CAD build for the part. Positions are in the model's coordinates, mm. Face numbers are marked on the shaded views. A direction names the side the tool comes from. Give positions to 0.01 mm unless a question says otherwise; leave off trailing zeros. Order: outer loops, then holes, each group sorted by start corner. A loop starts at its lowest first (then second) coordinate and runs counter-clockwise, first axis right, second up.
from build123d import *

# Parameters (mm, degrees)
F0_W     = 30
F0_H     = 50
F0_W_2   = 24
F0_H_2   = 44
F1_DEPTH = 250
F3_D     = 5.5
F5_D     = 10
F5_DEPTH = 5


with BuildPart() as f1:
    # F0 (on Top) → F1 (new body)
    with BuildSketch(Plane.XY):
        with Locations((15, 25)):
            Rectangle(F0_W, F0_H)
        with Locations((15, 25)):
            Rectangle(F0_W_2, F0_H_2, mode=Mode.SUBTRACT)
    extrude(amount=F1_DEPTH)

    # F3 (through all)
    with Locations(Plane(origin=(0, 0, 0), x_dir=(0, -1, 0), z_dir=(-1, 0, 0))):
        with Locations((-25, 220)):
            Hole(F3_D / 2)

    # F5
    with Locations(Plane.YZ.offset(30)):
        with Locations((25, 220)):
            Hole(F5_D / 2, depth=F5_DEPTH)


solid = f1.part
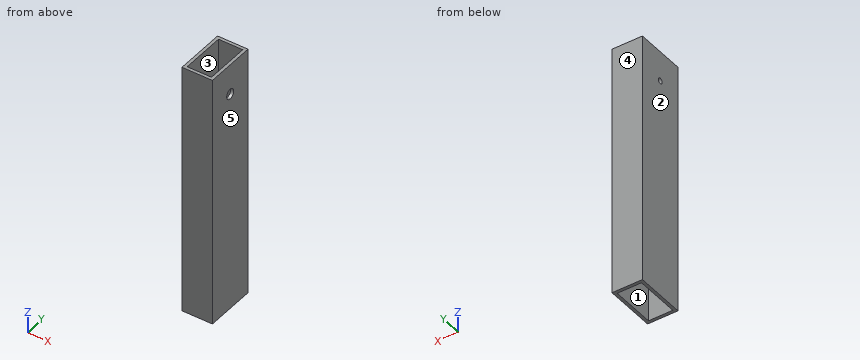
1. 3-axis set-ups, long thin cutter, end or side, ignore diameter. For the marked faces 1 and 2: which of +Z, -Z, +X, -X, +Y, -Y reach the whole face in a straight line?
2. Saw through at B-B on y = 44. Give the cut face in (x, z).
3. Saw through at A-A on x = 23.75. Give the cut face in (y, z), plus the area to 3 significant figures.
4. Mould opens along X. For the marked faces 3, 4 and 5 say: released by +X, released by -X, zero draft, split by the parting line, or undercut.
5. Saw through at C-C on z = 220. Give the cut face in (x, y), plus the area to 4 significant figures.
6. Wall check: line 1 (Z direction, x = 27.8, y = 25); line 2 (Y direction, x = 7.5, z = 87); line 3 (Z direction, x = 2.1, y = 25). Give the ranges that are in metal, low to high.
7. Saw through at D-D on y = 25. Give the cut face in (x, z).
Reported:
1. face 1: +Z, -Z
1. face 2: +Z, -Z, -X, +Y, -Y
2. outline: (0, 0) - (3, 0) - (3, 250) - (0, 250) - close; (27, 0) - (30, 0) - (30, 250) - (27, 250) - close
3. outline: (0, 0) - (3, 0) - (3, 250) - (0, 250) - close; (47, 0) - (50, 0) - (50, 250) - (47, 250) - close
3. area: 1,500 mm2
4. face 3: undercut
4. face 4: zero draft
4. face 5: released by +X
5. outline: (0, 0) - (30, 0) - (30, 20) - (27, 20) - (27, 3) - (3, 3) - (3, 22.25) - (0, 22.25) - close; (0, 27.75) - (3, 27.75) - (3, 47) - (27, 47) - (27, 30) - (30, 30) - (30, 50) - (0, 50) - close
5. area: 397.5 mm2
6. line 1: z = 0 to 215, 225 to 250
6. line 2: y = 0 to 3, 47 to 50
6. line 3: z = 0 to 217.25, 222.75 to 250
7. outline: (0, 0) - (3, 0) - (3, 217.25) - (0, 217.25) - close; (0, 222.75) - (3, 222.75) - (3, 250) - (0, 250) - close; (27, 0) - (30, 0) - (30, 215) - (27, 215) - close; (27, 225) - (30, 225) - (30, 250) - (27, 250) - close
